Could you check a few things on this model? Use its own coordinates, in mm. Give positions to 0.01 mm unless a question says otherwise; leave off trailing zeros. Loops run counter-clockwise (first coordinate to the right, second up) from the corner with the lowest first, then second, coordinate; pieces in that order, holes last. Notation, with made-up numbers: M -19.5,-13.5 L 22.5,-13.5 A21 cw 22.5,12.5 Z; hole C -14,52 d3. An arc over 180 degrees is marked long. Use a Markdown table: item, result. Add a question column.
1) Will these pins go through, and if not, where does the flat tip stop? pin 1 Ø3.5 at (x, y) = (32, 32) entering from -Z; pin 2 Ø1.5 at (y, z) = (1.5, 0.5) entering from -X.
2) Suppose I cut it at A-A on x = 47.5. List the corners of the cut face in (y, z) for me.
3) If I drill on line 1 along Y through (x, z) = (-31, 1.8); line 2 along Y through (x, z) = (32, 1.6); line 3 along X through (y, z) = (31.25, 1.55), over which ranges is the centre line in solid material (lowest first)? Write a range as [from, to].
4) Suppose I cut it at C-C on y = 47.5. List the corners of the cut face in (x, z) for me, and give its area (3 significant figures).
5) Suppose I cut it at B-B on z = 2.2. Count the separate pieces of the cut face and the enclosed holes in it, and give its area (3 significant figures).
Autodesk Inventor part; units mm, degrees
ref_plane "YZ Plane" through (0, 0, 0) normal (1, 0, 0) x (0, 1, 0)
ref_plane "XZ Plane" through (0, 0, 0) normal (0, 1, 0) x (-1, 0, 0)
ref_plane "XY Plane" through (0, 0, 0) normal (0, 0, 1) x (1, 0, 0)
sketch "Sketch3" plane through (0, 0, 0) normal (0, 0, 1) x (1, 0, 0)
  line L0 (50.9998, -51.0001) -> (-50.9998, -51.0001)
  line L1 (-50.9998, -51.0001) -> (-50.9998, 51.0001)
  line L2 (-50.9998, 51.0001) -> (50.9998, 51.0001)
  line L3 (50.9998, 51.0001) -> (50.9998, -51.0001)
  line L4 (50.9998, -51.0001) -> (-50.9998, 51.0001) construction
  line L5 (-50.9998, -51.0001) -> (50.9998, 51.0001) construction
  point P0 (0, 0)
  dimension "d2" = 101.9996
  dimension "d3" = 102.0002
sketch "Sketch7" plane through (0, 0, 0) normal (0, 0, 1) x (1, 0, 0)
  circle A0 centre (32.0004, 32.0005) radius 1.5002
  circle A1 centre (-31.9991, 32.0005) radius 1.5002
  circle A2 centre (-31.999, 32.0005) radius 1.5002
  circle A3 centre (-31.9991, -32.0002) radius 1.5002
  circle A4 centre (-31.999, -32.0002) radius 1.5002
  circle A5 centre (32.0003, -32.0002) radius 1.5002
  circle A6 centre (32.0004, -32.0002) radius 1.5002
extrude "Extrusion2" add sketch "Sketch3" along normal blind 3
hole "Hole1" at (-31.999, -32.0002, 0) at (-31.999, 32.0005, 0) at (32.0004, 32.0005, 0) at (32.0004, -32.0002, 0) direction (0, 0, 1) diameter 3 end through all countersink diameter 3.0226 countersink angle 82
sketch "Sketch8" plane through (0, 0, 0) normal (0, 0, -1) x (-1, 0, 0)
  circle A0 centre (47.5, 31.25) radius 1.2502
  circle A1 centre (31.25, 47.5) radius 1.2502
  circle A2 centre (-47.5, -31.25) radius 1.2502
  circle A3 centre (-31.25, -47.5) radius 1.2502
  circle A4 centre (-47.5, 31.25) radius 1.2502
  circle A5 centre (-31.25, 47.5) radius 1.2502
  circle A6 centre (47.5, -31.25) radius 1.2502
  circle A7 centre (31.25, -47.5) radius 1.2502
hole "Hole2" at (47.5, -31.25, 0) at (31.25, -47.5, 0) at (-31.25, -47.5, 0) at (-47.5, -31.25, 0) at (47.5, 31.25, 0) at (31.25, 47.5, 0) at (-31.25, 47.5, 0) at (-47.5, 31.25, 0) direction (0, 0, 1) diameter 2.5 end through all countersink diameter 2.6 countersink angle 82
sketch "Sketch9" plane through (0, 0, 0) normal (0, 0, -1) x (-1, 0, 0)
  point P0 (0, 0)
sketch "Sketch10" plane through (0, 0, 0) normal (0, 0, -1) x (-1, 0, 0)
  point P0 (0, 0)
sketch "Sketch11" plane through (0, 0, 0) normal (0, 0, -1) x (-1, 0, 0)
  line L0 (68.6779, 50.7734) -> (50.9999, 33.0954)
  line L1 (50.9999, 33.0954) -> (33.3221, 50.7732)
  line L2 (33.3221, 50.7732) -> (51.0001, 68.4512)
  line L3 (51.0001, 68.4512) -> (68.6779, 50.7734)
  line L4 (68.6779, 50.7734) -> (33.3221, 50.7732) construction
  line L5 (50.9999, 33.0954) -> (51.0001, 68.4512) construction
  line L6 (-33.3221, 50.7734) -> (-51.0001, 33.0954)
  line L7 (-51.0001, 33.0954) -> (-68.6779, 50.7732)
  line L8 (-68.6779, 50.7732) -> (-50.9999, 68.4512)
  line L9 (-50.9999, 68.4512) -> (-33.3221, 50.7734)
  line L10 (-33.3221, 50.7734) -> (-68.6779, 50.7732) construction
  line L11 (-51.0001, 33.0954) -> (-50.9999, 68.4512) construction
  line L12 (-33.3221, -51.2266) -> (-51.0001, -68.9046)
  line L13 (-51.0001, -68.9046) -> (-68.6779, -51.2268)
  line L14 (-68.6779, -51.2268) -> (-50.9999, -33.5488)
  line L15 (-50.9999, -33.5488) -> (-33.3221, -51.2266)
  line L16 (-33.3221, -51.2266) -> (-68.6779, -51.2268) construction
  line L17 (-51.0001, -68.9046) -> (-50.9999, -33.5488) construction
  line L18 (68.6779, -51.2266) -> (50.9999, -68.9046)
  line L19 (50.9999, -68.9046) -> (33.3221, -51.2268)
  line L20 (33.3221, -51.2268) -> (51.0001, -33.5488)
  line L21 (51.0001, -33.5488) -> (68.6779, -51.2266)
  line L22 (68.6779, -51.2266) -> (33.3221, -51.2268) construction
  line L23 (50.9999, -68.9046) -> (51.0001, -33.5488) construction
  point P0 (51, 50.7733)
  point P1 (-51, 50.7733)
  point P2 (-51, -51.2267)
  point P3 (51, -51.2267)
extrude "Extrusion3" cut sketch "Sketch11" against normal blind 3
sketch "Sketch12" plane through (0, 0, 0) normal (0, 0, -1) x (-1, 0, 0)
  line L0 (-50.9998, -33.5489) -> (-50.9998, 33.0957)
  arc A0 (-50.9998, -22.9999) -> (-50.9998, 22.9999) centre (-92.056, 0) ccw
  line L1 (-50.9998, 22.9999) -> (-50.9998, -22.9999)
  arc A1 (51.0009, 22.9999) -> (51.0009, -22.9999) centre (92.0571, 0) ccw
  line L2 (51.0009, -22.9999) -> (51.0009, 22.9999)
  point P0 (0, 0)
extrude "Extrusion4" cut sketch "Sketch12" against normal blind 3
properties part number "F450_GPS_mount." material "CFRP"
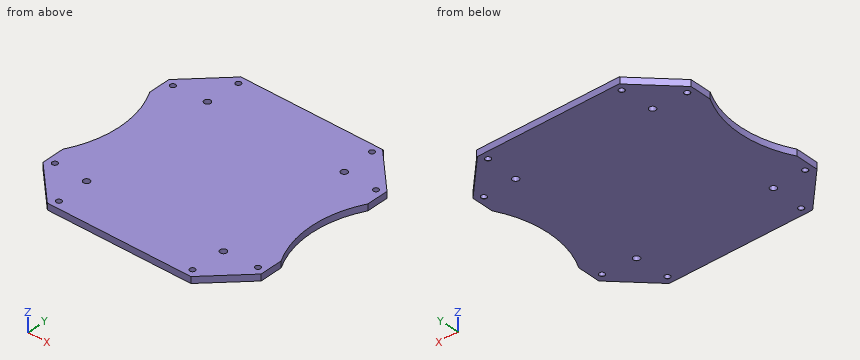
Answer block:
| question | item | result |
|---|---|---|
| 1 | pin 1 | stops at z = 0 |
| 1 | pin 2 | stops at x = -45.05 |
| 2 | outline | M -37.05,0 L -32.55,0 L -32.5,0.06 L -32.5,3 L -37.05,3 Z; M -30,0.06 L -29.95,0 L -15.14,0 L -15.14,3 L -30,3 Z; M 15.14,0 L 29.95,0 L 30,0.06 L 30,3 L 15.14,3 Z; M 32.5,0.06 L 32.55,0 L 36.6,0 L 36.6,3 L 32.5,3 Z |
| 3 | line 1 | y = [-51, -48.72], [-46.28, -33.12], [-30.88, 30.88], [33.12, 46.28], [48.72, 51] |
| 3 | line 2 | y = [-51, -48.5], [-46.5, -33.5], [-30.5, 30.5], [33.5, 46.5], [48.5, 51] |
| 3 | line 3 | x = [-51, -48.75], [-46.25, -33.3], [-30.7, 30.7], [33.3, 46.25], [48.75, 51] |
| 4 | outline | M -36.6,0 L -32.55,0 L -32.5,0.06 L -32.5,3 L -36.6,3 Z; M -30,0.06 L -29.95,0 L 29.95,0 L 30,0.06 L 30,3 L -30,3 Z; M 32.5,0.06 L 32.55,0 L 36.6,0 L 36.6,3 L 32.5,3 Z |
| 4 | area | 205 mm^2 |
| 5 | separate pieces | 1 |
| 5 | enclosed holes | 12 |
| 5 | area | 9,340 mm^2 |
